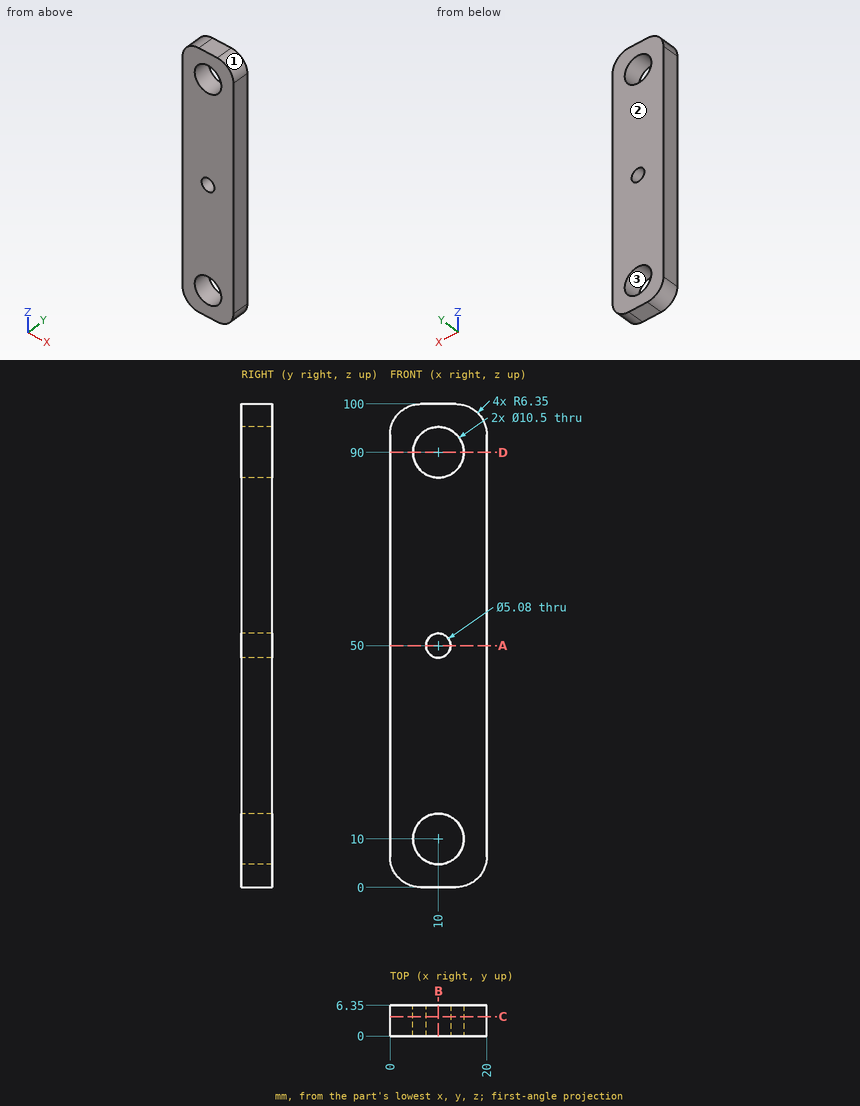
The figure shows three views and two pictorial views of one solid part (mm, origin at its lowest corner). Answer the questions. Round coordinates to 2 decimals unless told otherwise and drop trailing zeros. Write each loop counter-clockwise with the first axis right and the second up, starting at its lowest first coordinate (ties: lowest second). Pieces come first, ordered by that corner, then holes. Notation, with made-up numbers: (60, 88) - (117, 88) arc R16 cw to (117, 114) - close; hole circle Ø10 at (36.25, 10.25). An arc over 180 degrees is marked (long way). One line per question, with ' | ' between items. Start each with the question number.
1. This flat-tipped pin is pushed along its axis until it touches: pin 1 (5 mm diameter, centred on x = 9, z = 90, fed in from -Y). Where does it stop, or does it pass through?
2. Section D-D (z = 90) is taken. Determine the outline of the cut face in (x, y), and give its area (3 significant figures).
3. Section C-C (y = 4) is taken. Determine the outline of the cut face in (x, z).
4. Section A-A (z = 50) is taken. Determine the outline of the cut face in (x, y).
5. For a pull along X with two mould halves and no side action, classify the marked faces 1, 2 and 3 as +X half, -X half, draft (parallel to the pull), parting line (faces both ways), or undercut.
6. Find the intervals of material crossed by probe 1 along Z at (x, y) = (10, 3); probe 2 along X at (y, z) = (3.25, 90); probe 3 along Z at (x, y) = (8, 4.25), in increasing order. Write a range as [from, to].
7. Section B-B (x = 10) is taken. Determine the outline of the cut face in (y, z).
Filled in:
1) pin 1: through
2) outline: (0, 0) - (4.75, 0) - (4.75, 6.35) - (0, 6.35) - close; (15.25, 0) - (20, 0) - (20, 6.35) - (15.25, 6.35) - close | area: 60.3 mm²
3) outline: (0, 6.35) arc R6.35 ccw to (6.35, 0) - (13.65, 0) arc R6.35 ccw to (20, 6.35) - (20, 93.65) arc R6.35 ccw to (13.65, 100) - (6.35, 100) arc R6.35 ccw to (0, 93.65) - close; hole circle Ø10.5 at (10, 10); hole circle Ø10.5 at (10, 90); hole circle Ø5.08 at (10, 50)
4) outline: (0, 0) - (7.46, 0) - (7.46, 6.35) - (0, 6.35) - close; (12.54, 0) - (20, 0) - (20, 6.35) - (12.54, 6.35) - close
5) face 1: +X half | face 2: draft | face 3: undercut
6) probe 1: [0, 4.75], [15.25, 47.46], [52.54, 84.75], [95.25, 100] | probe 2: [0, 4.75], [15.25, 20] | probe 3: [0, 5.15], [14.85, 48.43], [51.57, 85.15], [94.85, 100]
7) outline: (0, 0) - (6.35, 0) - (6.35, 4.75) - (0, 4.75) - close; (0, 15.25) - (6.35, 15.25) - (6.35, 47.46) - (0, 47.46) - close; (0, 52.54) - (6.35, 52.54) - (6.35, 84.75) - (0, 84.75) - close; (0, 95.25) - (6.35, 95.25) - (6.35, 100) - (0, 100) - close
